```python
from build123d import *

# Parameters (mm, degrees)
BOSS_EXTRUDE1_DEPTH = 20
CUT_EXTRUDE2_REACH  = 39.964
SKETCH4_R           = 2.75
SKETCH2_R           = 4.75
CUT_EXTRUDE3_DEPTH  = 11.2
CUT_EXTRUDE4_REACH  = 39.964
SKETCH5_R           = 3
SKETCH6_R           = 5.5
CUT_EXTRUDE5_DEPTH  = 3.5
CHAMFER1_SIZE       = 0.5


with BuildPart() as part:
    # Sketch1 → Boss-Extrude1 (new body)
    with BuildSketch(Plane.XY):
        Polygon((-21, 0), (21, 0), (21, 20), (9, 20), (9, 24.5), (-9, 24.5), (-9, 20), (-21, 20), align=None)
    extrude(amount=-BOSS_EXTRUDE1_DEPTH)

    # Sketch4 → Cut-Extrude2 (cut, up to next)
    with BuildSketch(Plane(origin=(0, 0, 0), x_dir=(1, 0, 0), z_dir=(0, 1, 0)), mode=Mode.PRIVATE) as cut_extrude2_sk1:
        with Locations(Location((-15, 10, 0), (0, 0, 180))):
            Circle(SKETCH4_R)
    cut_extrude2_tool1 = extrude(cut_extrude2_sk1.sketch, amount=CUT_EXTRUDE2_REACH, mode=Mode.PRIVATE) & part.part
    cut_extrude2 = cut_extrude2_tool1.solids().sort_by_distance((-15, 0, -10))[0]
    add(cut_extrude2, mode=Mode.SUBTRACT)

    # Sketch2 → Cut-Extrude3 (cut)
    with BuildSketch(Plane(origin=(0, 20, 0), x_dir=(1, 0, 0), z_dir=(0, 1, 0))):
        with Locations(Location((-15, 10, 0), (0, 0, 270))):
            Circle(SKETCH2_R)
    cut_extrude3 = extrude(amount=-CUT_EXTRUDE3_DEPTH, mode=Mode.SUBTRACT)

    # Mirror1: Cut-Extrude2, Cut-Extrude3 across plane
    add(cut_extrude2.mirror(Plane(origin=(0, 0, 0), x_dir=(0, 0, 1), z_dir=(1, 0, 0))), mode=Mode.SUBTRACT)
    add(cut_extrude3.mirror(Plane(origin=(0, 0, 0), x_dir=(0, 0, 1), z_dir=(1, 0, 0))), mode=Mode.SUBTRACT)

    # Sketch5 → Cut-Extrude4 (cut, up to next)
    with BuildSketch(Plane.XY, mode=Mode.PRIVATE) as cut_extrude4_sk1:
        with Locations((0, 12.5)):
            Circle(SKETCH5_R)
    cut_extrude4_tool1 = extrude(cut_extrude4_sk1.sketch, amount=-CUT_EXTRUDE4_REACH, mode=Mode.PRIVATE) & part.part
    add(cut_extrude4_tool1.solids().sort_by_distance((0, 12.5, 0))[0], mode=Mode.SUBTRACT)

    # Sketch6 → Cut-Extrude5 (cut)
    with BuildSketch(Plane(origin=(0, 0, -20), x_dir=(-1, 0, 0), z_dir=(0, 0, -1))):
        with Locations((0, 12.5)):
            Circle(SKETCH6_R)
    extrude(amount=-CUT_EXTRUDE5_DEPTH, mode=Mode.SUBTRACT)

    # Chamfer1
    chamfer1_edges = [part.edges().sort_by_distance(p)[0] for p in [
        (0, 24.5, -20),
        (9, 22.25, 0),
        (15, 20, 0),
        (-9, 22.25, -20),
        (21, 20, -10),
        (21, 0, -10),
        (-21, 0, -10),
        (-21, 20, -10),
        (-9, 24.5, -10),
        (9, 24.5, -10),
        (-15, 20, -20),
        (-21, 10, -20),
        (0, 0, -20),
        (21, 10, -20),
        (15, 20, -20),
        (9, 22.25, -20),
        (21, 10, 0),
        (0, 0, 0),
        (-21, 10, 0),
        (-15, 20, 0),
        (-9, 22.25, 0),
        (0, 24.5, 0),
    ]]
    chamfer(chamfer1_edges, length=CHAMFER1_SIZE)


solid = part.part
```
For this review, take the finished solid that the model builds, in its own axes (mm). A direction names the side the tool comes from. Round coordinates to 2 decimals unless told otherwise and drop trailing zeros. Write each loop counter-clockwise with the first axis right and the second up, starting at its lowest first coordinate (ties: lowest second). Pieces come first, ordered by that corner, then holes. Notation, with made-up numbers: (-26, -18.5) - (17, -18.5) arc R24 ccw to (17, 19.5) - close; hole circle Ø7 at (41.5, -28.5). An arc over 180 degrees is marked (long way). Answer as a JSON object with one key per item and string values.
1. We need section C-C on z = -4. Give the boundary of the cut face in (x, y), then the cut area to 3 significant figures.
Response values:
{"outline": "(-21, 0.5) - (-20.5, 0) - (20.5, 0) - (21, 0.5) - (21, 19.5) - (20.5, 20) - (9, 20) - (9, 24) - (8.5, 24.5) - (-8.5, 24.5) - (-9, 24) - (-9, 20) - (-20.5, 20) - (-21, 19.5) - close; hole circle Ø6 at (0, 12.5)", "area": "892 mm2"}
2. We need section D-D on y = 3.25. Give the boundary of the cut face in (x, z), then the cut area to 3 significant figures.
Response values:
{"outline": "(-21, -19.5) - (-20.5, -20) - (20.5, -20) - (21, -19.5) - (21, -0.5) - (20.5, 0) - (-20.5, 0) - (-21, -0.5) - close; hole circle Ø5.5 at (-15, -10); hole circle Ø5.5 at (15, -10)", "area": "792 mm2"}
3. We need section B-B on x = 0. Give the boundary of the cut face in (y, z).
Response values:
{"outline": "(0, -19.5) - (0.5, -20) - (7, -20) - (7, -16.5) - (9.5, -16.5) - (9.5, 0) - (0.5, 0) - (0, -0.5) - close; (15.5, -16.5) - (18, -16.5) - (18, -20) - (24, -20) - (24.5, -19.5) - (24.5, -0.5) - (24, 0) - (15.5, 0) - close"}
4. For pin 1 Ø3 at (x, z) = (13.5, -9) entering from +Y; pin 2 Ø10 at (x, z) = (-14.5, -17.5) entering from +Y; pin 3 Ø1.2 at (y, z) = (21.5, -13.5) entering from +X, all flat-tipped, find the tip position at first contact; note any pin that passes through.
Response values:
{"pin 1": "stops at y = 8.8", "pin 2": "stops at y = 20", "pin 3": "stops at x = 9"}
5. To check wall thickness, follow line 1 along Y through (x, z) = (0, -18.25); line 2 along X through (y, z) = (16.25, -6); line 3 along X through (y, z) = (19.75, -9.5). State the ranges of each line that lie inside material, in increasing order.
Response values:
{"line 1": "y = 0 to 7, 18 to 24.5", "line 2": "x = -21 to -17.56, -12.44 to 12.44, 17.56 to 21", "line 3": "x = -20.75 to -19.72, -10.28 to 10.28, 19.72 to 20.75"}
6. Tool access review of faces 1 (the face through (1.19, 7.13, -18.27)), 2 (the face through (-12, 20, -6)), 3 (the face through (-13.57, 14.48, -5.47)), 4 (the face through (0, 7, 0)), 5 (the face through (12, 20, -6)): name each direction out of +Z, -Z, +X, -X, +Y, -Y from which nothing blocks a thin tool from reaching the whole face with its end or side.
Response values:
{"face 1": "-Z", "face 2": "+Z, -Z, -X, +Y", "face 3": "+Y", "face 4": "+Z, +X, -X, +Y, -Y", "face 5": "+Z, -Z, +X, +Y"}
7. Draft analysis for pull direction X (two halves, no side actions). For faces 6 (the face through (13.57, 14.48, -5.47)), 7 (the face through (-5, 7, -20)), 8 (the face through (9, 22, -10)), state which applies: +X half, -X half, draft (parallel to the pull), parting line (faces both ways), or undercut.
Response values:
{"face 6": "undercut", "face 7": "draft", "face 8": "+X half"}
8. We need section A-A on z = -10. Count the separate pieces of the cut face and the enclosed holes in it, then the cut area to 3 significant figures.
Response values:
{"separate pieces": "3", "enclosed holes": "1", "area": "582 mm2"}
